Could you check a few things on this model? Use its own coordinates, in mm. Face numbers are marked on the shaded views. Give positions to 0.01 mm unless a question says otherwise; leave off trailing zeros. Loops run counter-clockwise (first coordinate to the right, second up) from the corner with the lowest first, then second, coordinate; pieces in that order, holes last. Notation, with made-up numbers: M 24.25,-37.5 L 62.25,-37.5 A13 ccw 62.25,-13.5 Z; hole C 34,14 d10. An arc over 180 degrees is marked long. Return JSON: item names as keys, results as strings. Group by question number.
1. Please list where these lines run through material, in increasing order: line 1 (Y direction, x = -3.75, z = -5.5); line 2 (Y direction, x = -3.5, z = 9.5); line 3 (Z direction, x = -3.25, y = -7.5).
2. If we mould it in two halves opening along Z, with no side actions, what happens to the marked faces 1, 2 and 3? For each: +Z half, -Z half, draft (parallel to the pull), parting line (faces both ways), or undercut.
3. If we section it at B-B (z = 13.5): Write out the boundary of the cut face in (x, y), plus the area to 3 significant figures.
4. If we section it at D-D (z = 4.5): Write out the boundary of the cut face in (x, y), plus the area to 3 significant figures.
5. For pin 1 (4 mm diameter, centred on x = 2.5, y = -1, fed in from -Z); pin 2 (0.6 mm diameter, centred on y = 12, z = 11.5, fed in from +X); pin 3 (2.5 mm diameter, centred on x = 0.5, y = 1, fed in from +Z); pin 4 (5 mm diameter, centred on x = 2.5, y = -12, fed in from -Z), each with a flat end and sliding along its axis, tell me the tip position at first contact or that it passes through.
6. If we section it at A-A (y = 7.5): Write out the boundary of the cut face in (x, z).
7. If we section it at C-C (x = 1): Write out the boundary of the cut face in (y, z).
```python
from build123d import *

# Parameters (mm, degrees)
ESQUISSE3_W             = 40
ESQUISSE3_H             = 35.82
BOSS_EXTRU_1_DEPTH      = 2
ESQUISSE4_R             = 1
BOSS_EXTRU_2_DEPTH      = 2
ESQUISSE5_W             = 10.4
ESQUISSE5_H             = 2.9
ENL_V_MAT_EXTRU_1_DEPTH = 1
ESQUISSE6_W             = 12.4
ESQUISSE6_H             = 4.5
ENL_V_MAT_EXTRU_2_DEPTH = 1.5
ESQUISSE8_W             = 1.5
ESQUISSE8_H             = 6
BOSS_EXTRU_3_DEPTH      = 7
CONG_1_R                = 0.5
CONG_1_OF_SYM_TRIE1_R   = 0.5
CONG_2_R                = 3


with BuildPart() as part:
    # Esquisse3 → Boss.-Extru.1 (new body)
    with BuildSketch(Plane.ZY.offset(2.820074362)):
        Rectangle(ESQUISSE3_W, ESQUISSE3_H)
        Polygon((-13.98, 9.81), (-13.98, -9.69), (13.98, -9.69), (13.98, 9.81), (6, 9.81), (-6, 9.81), align=None, mode=Mode.SUBTRACT)
    extrude(amount=BOSS_EXTRU_1_DEPTH)

    # Esquisse4 → Boss.-Extru.2 (add)
    with BuildSketch(Plane(origin=(-2.820074362, 0, 0), x_dir=(0, 0, -1), z_dir=(1, 0, 0))):
        with Locations(Location((-11.668662175, 11.778743894, 0), (0, 0, 180))):
            Circle(ESQUISSE4_R)
        with Locations(Location((-11.668662175, -11.778743894, 0), (0, 0, 180))):
            Circle(ESQUISSE4_R)
        with Locations(Location((11.668662175, -11.778743894, 0), (0, 0, 180))):
            Circle(ESQUISSE4_R)
        with Locations(Location((11.668662175, 11.778743894, 0), (0, 0, 180))):
            Circle(ESQUISSE4_R)
    extrude(amount=BOSS_EXTRU_2_DEPTH)

    # Esquisse5 → Enlèv. mat.-Extru.1 (cut)
    with BuildSketch(Plane(origin=(-2.820074362, 0, 0), x_dir=(0, 0, -1), z_dir=(1, 0, 0))):
        with Locations((-0.22, -12.31)):
            Rectangle(ESQUISSE5_W, ESQUISSE5_H)
    extrude(amount=-ENL_V_MAT_EXTRU_1_DEPTH, mode=Mode.SUBTRACT)

    # Esquisse6 → Enlèv. mat.-Extru.2 (cut)
    with BuildSketch(Plane(origin=(-2.820074362, 0, 0), x_dir=(0, 0, -1), z_dir=(1, 0, 0))):
        with Locations((0, 11.86)):
            Rectangle(ESQUISSE6_W, ESQUISSE6_H)
    extrude(amount=-ENL_V_MAT_EXTRU_2_DEPTH, mode=Mode.SUBTRACT)

    # Esquisse8 → Boss.-Extru.3 (add)
    with BuildSketch(Plane(origin=(-2.820074362, 0, 0), x_dir=(0, 0, -1), z_dir=(1, 0, 0))):
        with Locations((-14.93, 0.06)):
            Rectangle(ESQUISSE8_W, ESQUISSE8_H)
    boss_extru_3 = extrude(amount=BOSS_EXTRU_3_DEPTH)

    # Congé1
    cong_1_edges = [part.edges().sort_by_distance(p)[0] for p in [
        (0.679925638, 3.06, 15.68),
        (0.679925638, -2.94, 15.68),
        (0.679925638, -2.94, 14.18),
        (0.679925638, 3.06, 14.18),
    ]]
    fillet(cong_1_edges, radius=CONG_1_R)

    # Symétrie1: Boss.-Extru.3 across plane
    add(boss_extru_3.mirror(Plane.XY))

    # Congé1 of Symétrie1
    cong_1_of_sym_trie1_edges = [part.edges().sort_by_distance(p)[0] for p in [
        (0.679925638, 3.06, -15.68),
        (0.679925638, -2.94, -15.68),
        (0.679925638, -2.94, -14.18),
        (0.679925638, 3.06, -14.18),
    ]]
    fillet(cong_1_of_sym_trie1_edges, radius=CONG_1_OF_SYM_TRIE1_R)

    # Congé2
    cong_2_edges = [part.edges().sort_by_distance(p)[0] for p in [
        (-3.820074362, 17.91, -20),
        (-3.820074362, 17.91, 20),
        (-3.820074362, -17.91, 20),
        (-3.820074362, -17.91, -20),
    ]]
    fillet(cong_2_edges, radius=CONG_2_R)


solid = part.part
```
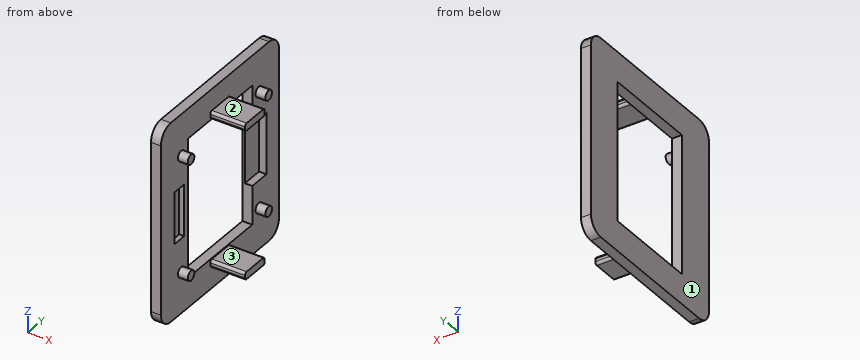
Answer:
{
 "1": {"line 1": "y = -17.91 to -9.69, 14.11 to 17.91", "line 2": "y = -17.91 to -9.69, 9.81 to 17.91", "line 3": "z = -20 to -13.98, 13.98 to 20"},
 "2": {"face 1": "draft", "face 2": "+Z half", "face 3": "undercut"},
 "3": {"outline": "M -4.82,-17.91 L -2.82,-17.91 L -2.82,-9.69 L -4.82,-9.69 Z; M -4.82,9.81 L -2.82,9.81 L -2.82,17.91 L -4.82,17.91 Z", "area": "32.6 mm²"},
 "4": {"outline": "M -4.82,-17.91 L -2.82,-17.91 L -2.82,-13.76 L -3.82,-13.76 L -3.82,-10.86 L -2.82,-10.86 L -2.82,-9.69 L -4.82,-9.69 Z; M -4.82,9.81 L -4.32,9.81 L -4.32,14.11 L -2.82,14.11 L -2.82,17.91 L -4.82,17.91 Z", "area": "23.3 mm²"},
 "5": {"pin 1": "stops at z = -15.68", "pin 2": "stops at x = -0.82", "pin 3": "stops at z = 15.68", "pin 4": "passes through"},
 "6": {"outline": "M -4.82,-20 L -2.82,-20 L -2.82,-13.98 L -4.82,-13.98 Z; M -4.82,13.98 L -2.82,13.98 L -2.82,20 L -4.82,20 Z"},
 "7": {"outline": "M -2.94,-15.18 A0.5 ccw -2.44,-15.68 L 2.56,-15.68 A0.5 ccw 3.06,-15.18 L 3.06,-14.68 A0.5 ccw 2.56,-14.18 L -2.44,-14.18 A0.5 ccw -2.94,-14.68 Z; M -2.94,14.68 A0.5 ccw -2.44,14.18 L 2.56,14.18 A0.5 ccw 3.06,14.68 L 3.06,15.18 A0.5 ccw 2.56,15.68 L -2.44,15.68 A0.5 ccw -2.94,15.18 Z"}
}
